CAD build for the part. Positions are in the model's coordinates, mm. Face numbers are marked on the shaded views. Coordinates: 2 decimals unless noted, no trailing zeros. Loops run counter-clockwise (first coordinate to the right, second up) from the corner with the lowest first, then second, coordinate; pieces in that order, holes last. Notation, with made-up numbers: (-19.75, 60.5) -> (-0.75, 60.5) arc R26 cw to (-0.75, 89.5) -> close; hole circle Ø6 at (-37.75, -17.75). An arc over 180 degrees is marked (long way). Write item = value, one per line. Start each with the question number.
(1) Pull direction Z, two halves, no side cores. Call the marked faces 1, 2 and 3: +Z half, -Z half, draft (parallel to the pull), parting line (faces both ways), or undercut.
(2) Band-saw the part on B-B (y = 4.5). Write the cut outline in (x, z), and give its area (3 significant figures).
(3) Drill centre lines: line 1 (Z direction, x = 16.5, y = 4); line 2 (Z direction, x = 6.5, y = 9); line 3 (Z direction, x = 3, y = 6.5). Where is each one in solid material? Low to high. Write a range as from..to.
(4) Flat gauge pins, fed straight in: P1, Ø12, axis at x = -1.5, z = -19, coming from the +Y side; P2, Ø2.5, axis at x = 16.5, z = -36.5, coming from the +Y side; P3, Ø20.5, axis at x = -5, z = 13.5, coming from the +Y side. Where does each tip first touch, or does it go through?
(5) Band-saw the part on D-D (z = 16). Write the cut outline in (x, y), and give its area (3 significant figures).
```python
from build123d import *

# Parameters (mm, degrees)
BOSS_EXTRUDE1_DEPTH        = 12
CUT_EXTRUDE1_DEPTH         = 4
SKETCH3_R                  = 7.75
CUT_EXTRUDE2_DEPTH         = 50.563091106
CUT_EXTRUDE3_DEPTH         = 49.595267259
CUT_EXTRUDE4_DEPTH         = 50.221438419
F_4_2_4_2_DIAMETER_HOLE1_D = 4.2
FILLET1_R                  = 1.5
FILLET2_R                  = 1.5


with BuildPart() as part:
    # Sketch1 → Boss-Extrude1 (new body)
    with BuildSketch(Plane(origin=(0, 0, 0), x_dir=(1, 0, 0), z_dir=(0, 1, 0))):
        with BuildLine():
            Line((-16.5, -42.5), (16.5, -42.5))
            ThreePointArc((16.5, -42.5), (20.742640687, -40.742640687), (22.5, -36.5))
            Line((22.5, -36.5), (22.5, 36.5))
            ThreePointArc((22.5, 36.5), (20.742640687, 40.742640687), (16.5, 42.5))
            Line((16.5, 42.5), (-16.5, 42.5))
            ThreePointArc((-16.5, 42.5), (-20.742640687, 40.742640687), (-22.5, 36.5))
            Line((-22.5, 36.5), (-22.5, -36.5))
            ThreePointArc((-22.5, -36.5), (-20.742640687, -40.742640687), (-16.5, -42.5))
        make_face()
    extrude(amount=BOSS_EXTRUDE1_DEPTH)

    # Sketch2 → Cut-Extrude1 (cut)
    with BuildSketch(Plane(origin=(0, 12, 0), x_dir=(1, 0, 0), z_dir=(0, 1, 0))):
        with BuildLine():
            Line((-16.5, -40.5), (16.5, -40.5))
            ThreePointArc((16.5, -40.5), (19.328427125, -39.328427125), (20.5, -36.5))
            Line((20.5, -36.5), (20.5, 36.5))
            ThreePointArc((20.5, 36.5), (19.328427125, 39.328427125), (16.5, 40.5))
            Line((16.5, 40.5), (-16.5, 40.5))
            ThreePointArc((-16.5, 40.5), (-19.328427125, 39.328427125), (-20.5, 36.5))
            Line((-20.5, 36.5), (-20.5, -36.5))
            ThreePointArc((-20.5, -36.5), (-19.328427125, -39.328427125), (-16.5, -40.5))
        make_face()
    extrude(amount=-CUT_EXTRUDE1_DEPTH, mode=Mode.SUBTRACT)

    # Sketch3 → Cut-Extrude2 (cut, through all)
    with BuildSketch(Plane(origin=(0, 0, 0), x_dir=(1, 0, 0), z_dir=(0, 1, 0))):
        with Locations(Location((0, 0, 0), (0, 0, 270))):
            Circle(SKETCH3_R)
    extrude(amount=CUT_EXTRUDE2_DEPTH, mode=Mode.SUBTRACT)

    # Sketch4 → Cut-Extrude3 (cut, through all)
    with BuildSketch(Plane(origin=(0, 7, 0), x_dir=(1, 0, 0), z_dir=(0, 1, 0))):
        with BuildLine():
            Line((-16, -30), (-16, 30))
            ThreePointArc((-16, 30), (-14.535533906, 33.535533906), (-11, 35))
            Line((-11, 35), (11, 35))
            ThreePointArc((11, 35), (14.535533906, 33.535533906), (16, 30))
            Line((16, 30), (16, -30))
            ThreePointArc((16, -30), (14.535533906, -33.535533906), (11, -35))
            Line((11, -35), (-11, -35))
            ThreePointArc((-11, -35), (-14.535533906, -33.535533906), (-16, -30))
        make_face()
    extrude(amount=CUT_EXTRUDE3_DEPTH, mode=Mode.SUBTRACT)

    # Sketch6 → Cut-Extrude4 (cut, through all)
    with BuildSketch(Plane(origin=(0, 1.5, 0), x_dir=(1, 0, 0), z_dir=(0, 1, 0))):
        with BuildLine():
            Line((-11, -34), (11, -34))
            ThreePointArc((11, -34), (13.828427125, -32.828427125), (15, -30))
            Line((15, -30), (15, 30))
            ThreePointArc((15, 30), (13.828427125, 32.828427125), (11, 34))
            Line((11, 34), (-11, 34))
            ThreePointArc((-11, 34), (-13.828427125, 32.828427125), (-15, 30))
            Line((-15, 30), (-15, -30))
            ThreePointArc((-15, -30), (-13.828427125, -32.828427125), (-11, -34))
        make_face()
    extrude(amount=CUT_EXTRUDE4_DEPTH, mode=Mode.SUBTRACT)

    # Ø4.2 (4.2) Diameter Hole1 (through all)
    with Locations(Plane.XZ):
        with Locations((-16.5, 36.5), (16.5, 36.5), (16.5, -36.5), (-16.5, -36.5)):
            Hole(F_4_2_4_2_DIAMETER_HOLE1_D / 2)

    # Fillet1
    fillet1_edges = [part.edges().sort_by_distance(p)[0] for p in [
        (20.742640687, 12, 40.742640687),
        (22.5, 12, 0),
        (20.742640687, 12, -40.742640687),
        (0, 12, -42.5),
        (-20.742640687, 12, -40.742640687),
        (-22.5, 12, 0),
        (-20.742640687, 12, 40.742640687),
        (0, 12, 42.5),
    ]]
    fillet(fillet1_edges, radius=FILLET1_R)

    # Fillet2
    fillet2_edges = [part.edges().sort_by_distance(p)[0] for p in [
        (0, 1.5, -7.75),
        (-13.828427125, 1.5, 32.828427125),
        (0, 1.5, 34),
        (13.828427125, 1.5, 32.828427125),
        (15, 1.5, 0),
        (13.828427125, 1.5, -32.828427125),
        (0, 1.5, -34),
        (-13.828427125, 1.5, -32.828427125),
        (-15, 1.5, 0),
    ]]
    fillet(fillet2_edges, radius=FILLET2_R - 0.0001)  # a hair under: the kernel refuses the full size


solid = part.part
```
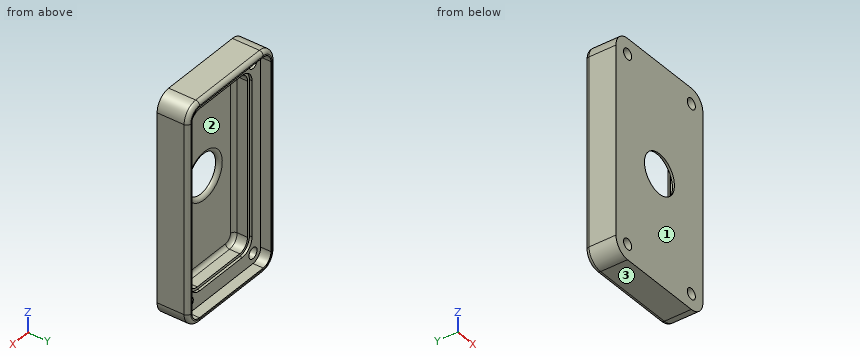
Findings below:
q1.face_1 = draft
q1.face_2 = undercut
q1.face_3 = -Z half
q2.outline = (-22.5, -36.5) arc R6 ccw to (-16.5, -42.5) -> (16.5, -42.5) arc R6 ccw to (22.5, -36.5) -> (22.5, 36.5) arc R6 ccw to (16.5, 42.5) -> (-16.5, 42.5) arc R6 ccw to (-22.5, 36.5) -> close; hole circle Ø4.2 at (-16.5, -36.5); hole circle Ø4.2 at (-16.5, 36.5); hole (-15, -30) arc R4 ccw to (-11, -34) -> (11, -34) arc R4 ccw to (15, -30) -> (15, 30) arc R4 ccw to (11, 34) -> (-11, 34) arc R4 ccw to (-15, 30) -> close; hole circle Ø4.2 at (16.5, -36.5); hole circle Ø4.2 at (16.5, 36.5)
q2.area = 1,710 mm²
q3.line_1 = -42.5..-38.6, -34.4..34.4, 38.6..42.5
q3.line_2 = -42.5..-40.5, 40.5..42.5
q3.line_3 = -42.5..-34, 34..42.5
q4.P1 = 1.5
q4.P2 = through
q4.P3 = 7
q5.outline = (-22.5, 0) -> (22.5, 0) -> (22.5, 10.5) arc R1.5 ccw to (21, 12) -> (20.5, 12) -> (20.5, 8) -> (16, 8) -> (16, 7) -> (15, 7) -> (15, 3) arc R1.5 cw to (13.5, 1.5) -> (-13.5, 1.5) arc R1.5 cw to (-15, 3) -> (-15, 7) -> (-16, 7) -> (-16, 8) -> (-20.5, 8) -> (-20.5, 12) -> (-21, 12) arc R1.5 ccw to (-22.5, 10.5) -> close
q5.area = 179 mm²
